The drawing under review shows one solid part. Ordinate dimensions are in mm from its lowest x, y, z. A direction names the side the tool comes from. Round coordinates to 2 decimals unless told otherwise and drop trailing zeros. Order: outer loops, then holes, each group sorted by start corner. A loop starts at its lowest first (then second) coordinate and runs counter-clockwise, first axis right, second up. Notation, with made-up numbers: M 69,18.5 L 114,18.5 A18 cw 114,41.5 Z; hole C 34.25,11 d1. An arc over 180 degrees is marked long. Answer as a JSON object with one key per item and string values. Group by question number.
1) To check wall thickness, follow line 1 (X direction, y = 8.75, z = 48) (1 decimal); line 2 (X direction, y = 3.75, z = 42) (1 decimal); line 3 (X direction, y = 8.5, z = 58) (1 decimal). State the ranges of each line that lie inside material, in increasing order.
2) Consider section A-A, the plane x = 5.5. Write out the cut boundary in (y, z).
3) Consider section D-D, the plane x = 62. Write out the cut boundary in (y, z) (1 decimal).
4) For the marked faces 5, 6, 7, 8 and 9, list the 3-axis set-ups (+Z, -Z, +X, -X, +Y, -Y) from which the entire face can be reached by the end or side of a thin tool; tool diameter is ignored.
5) Consider section C-C, the plane y = 2.75. Write out the cut boundary in (x, z) (1 decimal).
6) The part is to be moulded in two halves that separate along Z. For the marked faces 1, 2, 3 and 4, say which applies: +Z half, -Z half, draft (parallel to the pull), parting line (faces both ways), or undercut.
7) Consider section B-B, the plane z = 30.5. Write out the cut boundary in (x, y) (1 decimal), then the cut area to 3 significant figures.
8) Insertion check: pin 1 Ø11 at (x, z) = (27, 30.5) entering from +Y. The pin has a flat end and moves straight along its axis. Give the tip position at first contact, or say it passes through.
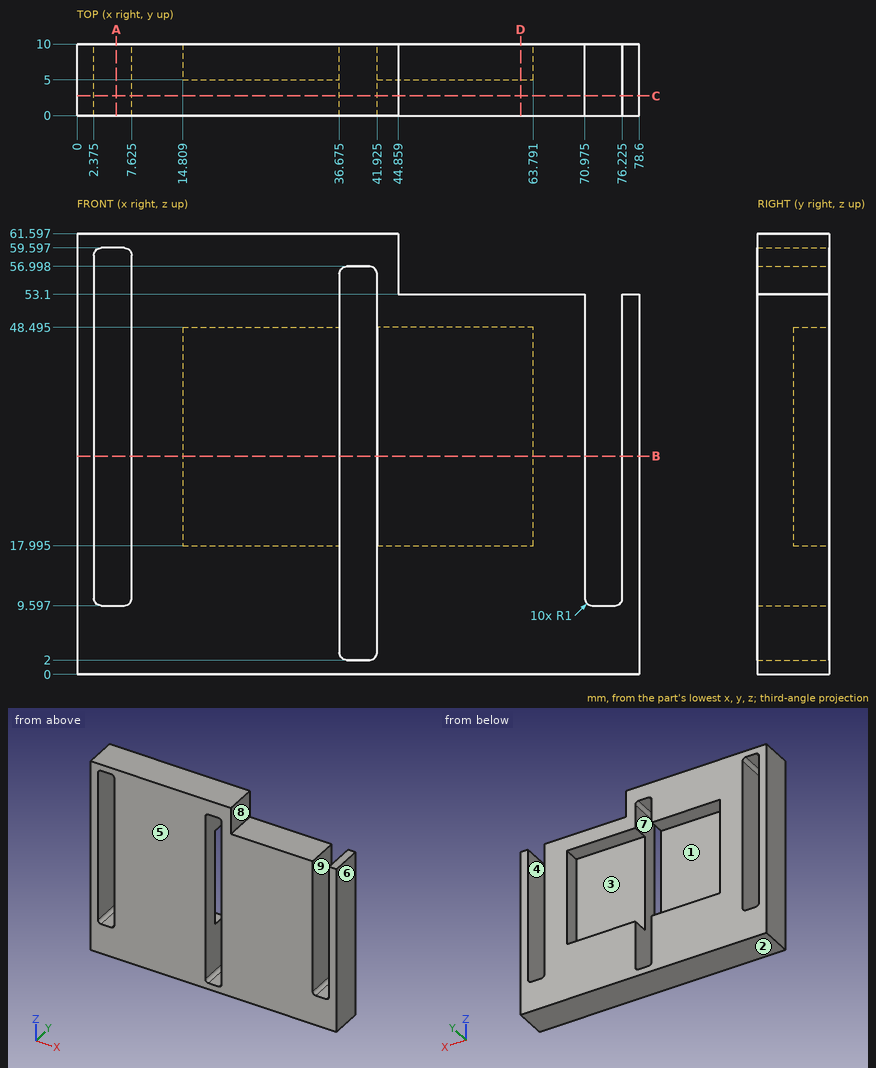
Results list:
{
 "1": {"line 1": "0 to 2.4, 7.6 to 14.8, 63.8 to 71, 76.2 to 78.6", "line 2": "0 to 2.4, 7.6 to 36.7, 41.9 to 71, 76.2 to 78.6", "line 3": "0 to 2.4, 7.6 to 44.9"},
 "2": {"outline": "M 0,0 L 10,0 L 10,9.6 L 0,9.6 Z; M 0,59.6 L 10,59.6 L 10,61.6 L 0,61.6 Z"},
 "3": {"outline": "M 0,0 L 10,0 L 10,18 L 5,18 L 5,48.5 L 10,48.5 L 10,53.1 L 0,53.1 Z"},
 "4": {"face 5": "+Z, -Z, +X, -X, -Y", "face 6": "+Z, -Z, +X, +Y, -Y", "face 7": "+Y, -Y", "face 8": "+Z, +X, +Y, -Y", "face 9": "+Z, +Y, -Y"},
 "5": {"outline": "M 0,0 L 78.6,0 L 78.6,53.1 L 76.2,53.1 L 76.2,10.6 A1 cw 75.2,9.6 L 72,9.6 A1 cw 71,10.6 L 71,53.1 L 44.9,53.1 L 44.9,61.6 L 0,61.6 Z; hole M 2.4,10.6 A1 ccw 3.4,9.6 L 6.6,9.6 A1 ccw 7.6,10.6 L 7.6,58.6 A1 ccw 6.6,59.6 L 3.4,59.6 A1 ccw 2.4,58.6 Z; hole M 36.7,3 A1 ccw 37.7,2 L 40.9,2 A1 ccw 41.9,3 L 41.9,56 A1 ccw 40.9,57 L 37.7,57 A1 ccw 36.7,56 Z"},
 "6": {"face 1": "undercut", "face 2": "-Z half", "face 3": "undercut", "face 4": "draft"},
 "7": {"outline": "M 0,0 L 2.4,0 L 2.4,10 L 0,10 Z; M 7.6,0 L 36.7,0 L 36.7,5 L 14.8,5 L 14.8,10 L 7.6,10 Z; M 41.9,0 L 71,0 L 71,10 L 63.8,10 L 63.8,5 L 41.9,5 Z; M 76.2,0 L 78.6,0 L 78.6,10 L 76.2,10 Z", "area": "410 mm^2"},
 "8": {"pin 1": "y = 5"}
}
